from build123d import *

# Parameters (mm, degrees)
SKETCH1_W           = 12.3698
SKETCH1_H           = 22.5552
BOSS_EXTRUDE1_DEPTH = 11.36015
BOSS_EXTRUDE2_DEPTH = 2.37
BOSS_EXTRUDE3_DEPTH = 4.31
SKETCH4_R           = 2.41
SKETCH4_R_2         = 0.75
BOSS_EXTRUDE4_DEPTH = 2.75


with BuildPart() as part:
    # Sketch1 → Boss-Extrude1 (new, symmetric)
    with BuildSketch(Plane.XY):
        Rectangle(SKETCH1_W, SKETCH1_H)
    extrude(amount=BOSS_EXTRUDE1_DEPTH, both=True)

    # Sketch2 → Boss-Extrude2 (add)
    with BuildSketch(Plane.XY.offset(7.10565)):
        with BuildLine():
            Line((-0.575, 16.0401), (-6.1849, 16.0401))
            Line((-6.1849, 16.0401), (-6.1849, 11.2776))
            Line((-6.1849, 11.2776), (6.1849, 11.2776))
            Line((6.1849, 11.2776), (6.1849, 16.0401))
            Line((6.1849, 16.0401), (0.575, 16.0401))
            Line((0.575, 16.0401), (0.575, 15.0401))
            ThreePointArc((0.575, 15.0401), (0, 12.1546849), (-0.575, 15.0401))
            Line((-0.575, 15.0401), (-0.575, 16.0401))
        make_face()
    boss_extrude2 = extrude(amount=-BOSS_EXTRUDE2_DEPTH)

    # Mirror1: Boss-Extrude2 across plane
    add(boss_extrude2.mirror(Plane.ZX))

    # Sketch3 → Boss-Extrude3 (add)
    with BuildSketch(Plane.XY.offset(11.36015)):
        with BuildLine():
            Line((2.7, -0.5224), (2.7, -0.471739595))
            ThreePointArc((2.7, -0.471739595), (0, 11.2776), (-2.7, -0.471739595))
            Line((-2.7, -0.471739595), (-2.7, -0.5224))
            ThreePointArc((-2.7, -0.5224), (0, -3.2224), (2.7, -0.5224))
        make_face()
    extrude(amount=BOSS_EXTRUDE3_DEPTH)

    # Sketch4 → Boss-Extrude4 (add)
    with BuildSketch(Plane.XY.offset(15.67015)):
        with Locations((0, 5.0927)):
            Circle(SKETCH4_R)
        with Locations((0, 5.0927)):
            Circle(SKETCH4_R_2, mode=Mode.SUBTRACT)
    extrude(amount=BOSS_EXTRUDE4_DEPTH)


solid = part.part
Verification items for the finished model (mm, model axes). A direction names the side the tool comes from. Coordinates: 2 decimals unless noted, no trailing zeros. Loops run counter-clockwise (first coordinate to the right, second up) from the corner with the lowest first, then second, coordinate; pieces in that order, holes last. Notation, with made-up numbers: (63.25, -28) -> (84.25, -28) arc R26 cw to (84.25, -3) -> close; hole circle Ø11 at (89.5, -3.5). An arc over 180 degrees is marked (long way). Answer as a JSON object with one key per item and string values. Group by question number.
Item 1: Sectioned sample at A-A on x = 4.75. Record the boundary of the cut face in (y, z).
Item 2: Scan lines: probe 1 along Y at (x, z) = (0, 16.6); probe 2 along Z at (x, y) = (-4.75, 7.5); probe 3 along Z at (x, y) = (3.5, 12). Record each from-to range of solid material in increasing order.
Item 3: Tool access check on faces 1 (the flat face through (0, -12, 7.106)), 2 (the cylindrical face through (-0.16, 4.36, 17.03)), 3 (the flat face through (0, -11.278, -3)), 4 (the flat face through (0.575, -15.5, 5.9)), 5 (the flat face through (0, 12, 4.736)). Record the directions out of +Z, -Z, +X, -X, +Y, -Y that give a thin tool (end or side, any length) a straight path to the whole face; none if there is none.
Item 4: Sectioned sample at D-D on y = -8. Record the boundary of the cut face in (x, z), plus the area to 3 significant figures.
Item 5: Sectioned sample at C-C on z = 15.25. Record the boundary of the cut face in (x, y), plus the area to 3 significant figures.
Item 6: Depth check by flat-ended pin: pin 1 (4 mm diameter, centred on x = 0, y = -13.5, fed in from +Z); pin 2 (3 mm diameter, centred on x = 2, y = 9.5, fed in from +Z); pin 3 (3.5 mm diameter, centred on x = 0.5, z = 10, fed in from +Y). Enter the tip coordinate at first touch or a pass-through.
Item 7: Sectioned sample at B-B on y = 8. Record the boundary of the cut face in (x, z).
Evaluation:
{
 "1": {"outline": "(-16.04, 4.74) -> (-11.28, 4.74) -> (-11.28, -11.36) -> (11.28, -11.36) -> (11.28, 4.74) -> (16.04, 4.74) -> (16.04, 7.11) -> (11.28, 7.11) -> (11.28, 11.36) -> (9.05, 11.36) -> (9.05, 15.67) -> (1.13, 15.67) -> (1.13, 11.36) -> (-11.28, 11.36) -> (-11.28, 7.11) -> (-16.04, 7.11) -> close"},
 "2": {"probe 1": "y = 2.68 to 4.34, 5.84 to 7.5", "probe 2": "z = -11.36 to 15.67", "probe 3": "z = 4.74 to 7.11"},
 "3": {"face 1": "+Z, +X, -X, -Y", "face 2": "+Z", "face 3": "-Z, +X, -X, -Y", "face 4": "+Z, -Z, -Y", "face 5": "-Z, +X, -X, +Y"},
 "4": {"outline": "(-6.18, -11.36) -> (6.18, -11.36) -> (6.18, 11.36) -> (-6.18, 11.36) -> close", "area": "281 mm²"},
 "5": {"outline": "(-2.7, -0.52) arc R2.7 ccw to (2.7, -0.52) -> (2.7, -0.47) arc R6.18 ccw (long way) to (-2.7, -0.47) -> close", "area": "130 mm²"},
 "6": {"pin 1": "stops at z = 7.11", "pin 2": "stops at z = 15.67", "pin 3": "stops at y = 11.28"},
 "7": {"outline": "(-6.18, -11.36) -> (6.18, -11.36) -> (6.18, 11.36) -> (5.46, 11.36) -> (5.46, 15.67) -> (-5.46, 15.67) -> (-5.46, 11.36) -> (-6.18, 11.36) -> close"}
}
